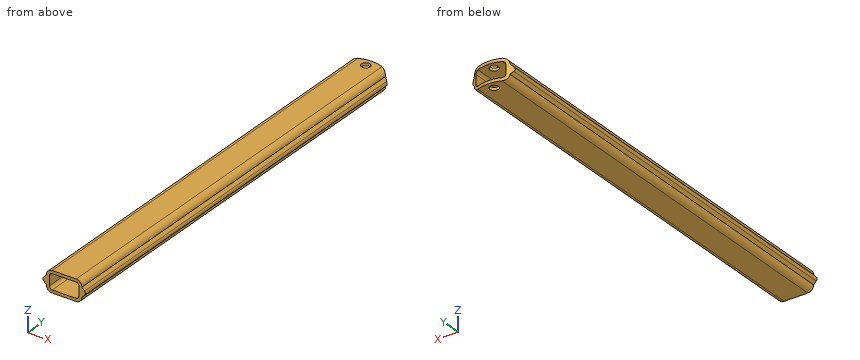
```python
from build123d import *

# Parameters (mm, degrees)
F1_DEPTH = 150
F2_R     = 1.5
F3_DEPTH = 7.301
F6_DEPTH = 25


# Not quite as in the source:
# - a feature names something its author has since deleted; it is built from what else it names


with BuildPart() as f1:
    # F0 (on Front) → F1 (new body)
    with BuildSketch(Plane.XZ):
        with BuildLine():
            Line((7.0581561667, 0.685534298), (6.15, 1.65))
            ThreePointArc((6.15, 1.65), (5.5642135624, 3.0642135624), (4.15, 3.65))
            Line((4.15, 3.65), (-4.15, 3.65))
            ThreePointArc((-4.15, 3.65), (-5.5642135624, 3.0642135624), (-6.15, 1.65))
            Line((-6.15, 1.65), (-7.0581561667, 0.685534298))
            ThreePointArc((-7.0581561667, 0.685534298), (-7.3301158338, 0), (-7.0581561667, -0.685534298))
            Line((-7.0581561667, -0.685534298), (-6.15, -1.65))
            ThreePointArc((-6.15, -1.65), (-5.5642135624, -3.0642135624), (-4.15, -3.65))
            Line((-4.15, -3.65), (4.15, -3.65))
            ThreePointArc((4.15, -3.65), (5.5642135624, -3.0642135624), (6.15, -1.65))
            Line((6.15, -1.65), (7.0581561667, -0.685534298))
            ThreePointArc((7.0581561667, -0.685534298), (7.3301158338, 0), (7.0581561667, 0.685534298))
        make_face()
        with BuildLine():
            ThreePointArc((5.15, -1.65), (4.8571067812, -2.3571067812), (4.15, -2.65))
            Line((4.15, -2.65), (-4.15, -2.65))
            ThreePointArc((-4.15, -2.65), (-4.8571067812, -2.3571067812), (-5.15, -1.65))
            Line((-5.15, -1.65), (-5.15, 1.65))
            ThreePointArc((-5.15, 1.65), (-4.8571067812, 2.3571067812), (-4.15, 2.65))
            Line((-4.15, 2.65), (4.15, 2.65))
            ThreePointArc((4.15, 2.65), (4.8571067812, 2.3571067812), (5.15, 1.65))
            Line((5.15, 1.65), (5.15, -1.65))
        make_face(mode=Mode.SUBTRACT)
    extrude(amount=F1_DEPTH)

    # F2 (on face) → F3 (cut, through all)
    with BuildSketch(Plane.XY.offset(3.65)):
        with Locations((0, -3)):
            Circle(F2_R)
    extrude(amount=-F3_DEPTH, mode=Mode.SUBTRACT)

    # F5 (on offset) → F6 (cut)
    with BuildSketch(Plane.XY.offset(4.6)):
        with BuildLine():
            Line((8, -3.7011680724), (8, 3.7011680724))
            Line((8, 3.7011680724), (-8, 3.7011680724))
            Line((-8, 3.7011680724), (-8, -3.7011680724))
            ThreePointArc((-8, -3.7011680724), (0, -0.1482238292), (8, -3.7011680724))
        make_face()
    extrude(amount=-F6_DEPTH, mode=Mode.SUBTRACT)


solid = f1.part
```
Verification items for the finished model (mm, model axes). Round coordinates to 2 decimals unless told otherwise and drop trailing zeros. Order: outer loops, then holes, each group sorted by start corner. A loop starts at its lowest first (then second) coordinate and runs counter-clockwise, first axis right, second up.
1) Depth check by flat-ended pin: pin 1 (3 mm diameter, centred on x = 3, z = -2, fed in from +Y). Enter the tip coordinate at first touch or a pass-through.
Geometry says:
pin 1: stops at y = -0.27
2) Cross-section at B-B, the plane y = -60. Record the cut outline in (x, z).
Geometry says:
outline: (-7.06, -0.69) - (-6.15, -1.65) arc R2 ccw to (-4.15, -3.65) - (4.15, -3.65) arc R2 ccw to (6.15, -1.65) - (7.06, -0.69) arc R1 ccw to (7.06, 0.69) - (6.15, 1.65) arc R2 ccw to (4.15, 3.65) - (-4.15, 3.65) arc R2 ccw to (-6.15, 1.65) - (-7.06, 0.69) arc R1 ccw to start; hole (-5.15, -1.65) arc R1 ccw to (-4.15, -2.65) - (4.15, -2.65) arc R1 ccw to (5.15, -1.65) - (5.15, 1.65) arc R1 ccw to (4.15, 2.65) - (-4.15, 2.65) arc R1 ccw to (-5.15, 1.65) - close
3) Cross-section at A-A, the plane x = 0. Record the cut outline in (y, z).
Geometry says:
outline: (-150, -3.65) - (-4.5, -3.65) - (-4.5, -2.65) - (-150, -2.65) - close; (-150, 2.65) - (-4.5, 2.65) - (-4.5, 3.65) - (-150, 3.65) - close; (-1.5, -3.65) - (-0.15, -3.65) - (-0.15, -2.65) - (-1.5, -2.65) - close; (-1.5, 2.65) - (-0.15, 2.65) - (-0.15, 3.65) - (-1.5, 3.65) - close
4) Material ranges on line 1 (Y direction, x = 0, z = -3.05); line 2 (Z direction, x = 2.25, y = -16); line 3 (X direction, y = -15.5, z = 0), recorded low to high.
Geometry says:
line 1: y = -150 to -4.5, -1.5 to -0.15
line 2: z = -3.65 to -2.65, 2.65 to 3.65
line 3: x = -7.33 to -5.15, 5.15 to 7.33
